Job drawing, mm, ordinate dimensions from the low corner. One solid piece. Give positions to 0.01 mm unless a question says otherwise; leave off trailing zeros. Loops run counter-clockwise (first coordinate to the right, second up) from the corner with the lowest first, then second, coordinate; pieces in that order, holes last. Notation, with made-up numbers: (62, 47) - (86, 47) arc R31 cw to (86, 80) - close; hole circle Ø4 at (-17.75, 13.25). An arc over 180 degrees is marked (long way). Use a Markdown table: item, result.
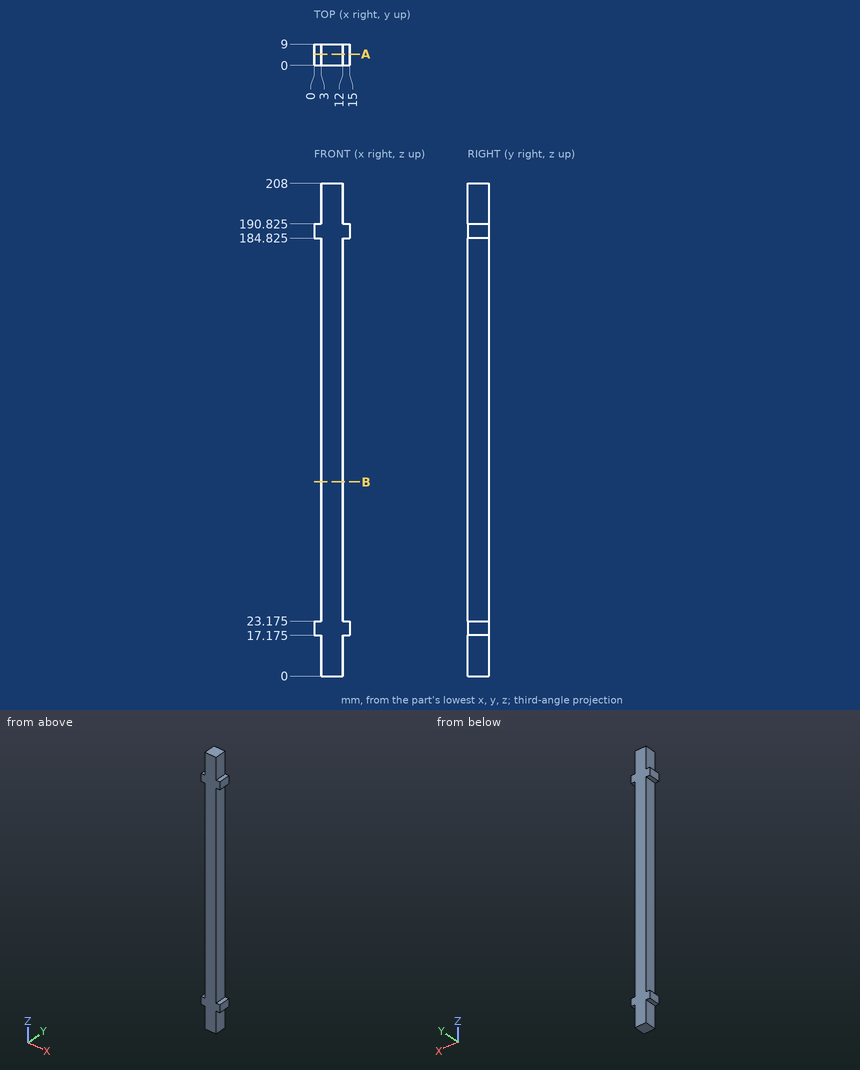
(1) Drill centre lines: probe 1 along Z at (x, y) = (2, 1.25) (3 decimals); probe 2 along X at (y, z) = (5.75, 144.5). Where is each one in solid material? Low to high. Write a range as [from, to].
Computed:
| item | result |
|---|---|
| probe 1 | [17.175, 23.175], [184.825, 190.825] |
| probe 2 | [3, 12] |
(2) Slice it at B-B, the plane z = 82. Write the cut outline in (x, y).
Computed:
| item | result |
|---|---|
| outline | (3, 0) - (12, 0) - (12, 9) - (3, 9) - close |
(3) Pin check, flat tips, straight feed: P1, Ø1.5, axis at x = 2, y = 2.5, coming from the +Z side (3 decimals); P2, Ø4.5, axis at y = 5.5, z = 6, coming from the -X side; P3, Ø1.5, axis at x = 1.5, y = 2.5, coming from the -Z side (3 decimals). Stop position of each tip, or through.
Computed:
| item | result |
|---|---|
| P1 | z = 190.825 |
| P2 | x = 3 |
| P3 | z = 17.175 |
(4) Slice it at A-A, the plane y = 4.75. Write the cut outline in (x, z) (3 decimals).
Computed:
| item | result |
|---|---|
| outline | (0, 17.175) - (3, 17.175) - (3, 0) - (12, 0) - (12, 17.175) - (15, 17.175) - (15, 23.175) - (12, 23.175) - (12, 184.825) - (15, 184.825) - (15, 190.825) - (12, 190.825) - (12, 208) - (3, 208) - (3, 190.825) - (0, 190.825) - (0, 184.825) - (3, 184.825) - (3, 23.175) - (0, 23.175) - close |
